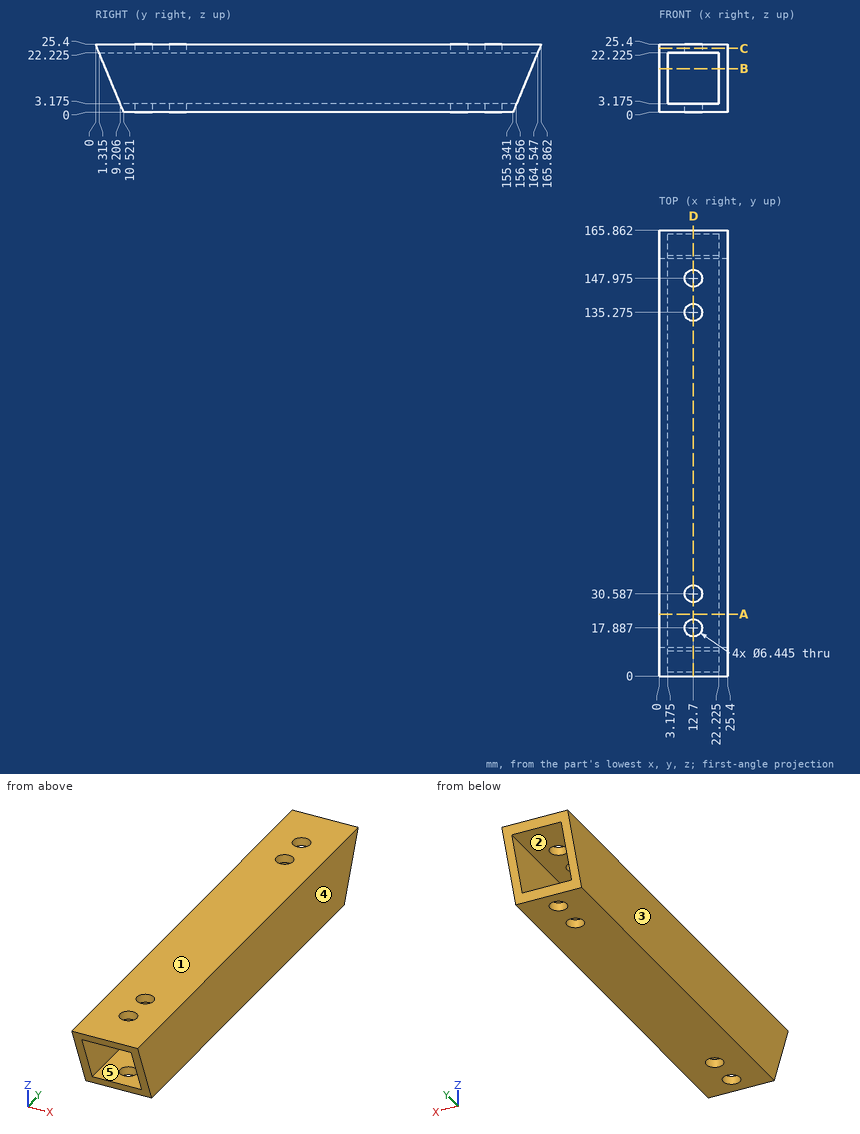
Job drawing, mm, ordinate dimensions from the low corner. One solid piece. A direction names the side the tool comes from. Give positions to 0.01 mm unless a question says otherwise; leave off trailing zeros. Loops run counter-clockwise (first coordinate to the right, second up) from the corner with the lowest first, then second, coordinate; pieces in that order, holes last. Notation, with made-up numbers: (4.5, -7) -> (27.5, -7) arc R15 ccw to (27.5, 10) -> close; hole circle Ø8 at (74, 40.5). An arc over 180 degrees is marked (long way). Use a Markdown table: item, result. Add a question column.
(1) Slice it at D-D on x = 12.7. Give the number of separate pieces and of enclosed holes in the cut face.
(2) Slice it at C-C on z = 23.75. List the corners of the cut face in (x, y) (1 decimal), and give its area (3 significant figures).
(3) Drop flat-ended pins along their axis: pin 1 Ø5 at (x, y) = (12.7, 30.59) entering from -Z; pin 2 Ø2 at (x, z) = (20, 3) entering from -Y. Give the stop position or say it passes through.
(4) Wall check: line 1 along X through (y, z) = (33, 17) (3 decimals); line 2 along Y through (x, z) = (12.7, 23.55) (1 decimal). Give the ranges that are in metal, low to high.
(5) Slice it at A-A on y = 23. List the corners of the cut face in (x, z) (3 decimals).
(6) Mould opens along Z. For the marked faces 1, 2 and 3 say: +Z half, -Z half, draft (parallel to the pull), parting line (faces both ways), or undercut.
(7) Tool access for the marked faces 4 and 5: list every direction of +Z, -Z, +X, -X, +Y, -Y with a clear straight run to the whole face (end or side of a thin tool).
(8) Slice it at B-B on z = 16.25. List the corners of the cut face in (x, y) (1 decimal).
Filled sheet:
| question | item | result |
|---|---|---|
| 1 | separate pieces | 10 |
| 1 | enclosed holes | 0 |
| 2 | outline | (0, 0.7) -> (25.4, 0.7) -> (25.4, 165.2) -> (0, 165.2) -> close; hole circle Ø6.4 at (12.7, 17.9); hole circle Ø6.4 at (12.7, 30.6); hole circle Ø6.4 at (12.7, 135.3); hole circle Ø6.4 at (12.7, 148) |
| 2 | area | 4,050 mm2 |
| 3 | pin 1 | through |
| 3 | pin 2 | y = 9.21 |
| 4 | line 1 | 0 to 3.175, 22.225 to 25.4 |
| 4 | line 2 | 0.8 to 14.7, 21.1 to 27.4, 33.8 to 132.1, 138.5 to 144.8, 151.2 to 165.1 |
| 5 | outline | (0, 0) -> (25.4, 0) -> (25.4, 25.4) -> (0, 25.4) -> close; hole (3.175, 3.175) -> (22.225, 3.175) -> (22.225, 22.225) -> (3.175, 22.225) -> close |
| 6 | face 1 | +Z half |
| 6 | face 2 | undercut |
| 6 | face 3 | draft |
| 7 | face 4 | +Z, -Z, +X, +Y, -Y |
| 7 | face 5 | +Y, -Y |
| 8 | outline | (0, 3.8) -> (3.2, 3.8) -> (3.2, 162.1) -> (0, 162.1) -> close; (22.2, 3.8) -> (25.4, 3.8) -> (25.4, 162.1) -> (22.2, 162.1) -> close |
